Part model, mm, in its own coordinate system. A direction names the side the tool comes from. Coordinates: 2 decimals unless noted, no trailing zeros. Loops run counter-clockwise (first coordinate to the right, second up) from the corner with the lowest first, then second, coordinate; pieces in that order, holes last. Notation, with made-up numbers: M 78,87.25 L 127,87.25 A22 cw 127,118.25 Z; hole C -4,64 d2. An arc over 180 degrees is marked long. Answer as CSV lines item,"result". Start each with the question number.
from build123d import *

# Parameters (mm, degrees)
SKETCH1_W                        = 38.1
SKETCH1_H                        = 19.05
BOSS_EXTRUDE1_DEPTH              = 27.94
SKETCH2_W                        = 8.89
SKETCH2_H                        = 19.05
CUT_EXTRUDE1_DEPTH               = 21.59
CUT_EXTRUDE2_DEPTH               = 31.75
F_43_0_089_DIAMETER_HOLE1_D      = 2.2606
F_51_0_067_DIAMETER_HOLE1_REACH  = 52.943
F_51_0_067_DIAMETER_HOLE1_BORE_R = 0.8509
FILLET1_R                        = 1.27
SKETCH11_R                       = 2.75
CUT_EXTRUDE3_DEPTH               = 2
SKETCH12_R                       = 2.159
SKETCH12_R_2                     = 2.1209
CUT_EXTRUDE4_DEPTH               = 2.54


with BuildPart() as part:
    # Sketch1 → Boss-Extrude1 (new body)
    with BuildSketch(Plane.XY):
        with Locations((19.05, 9.525)):
            Rectangle(SKETCH1_W, SKETCH1_H)
    extrude(amount=BOSS_EXTRUDE1_DEPTH)

    # Sketch2 → Cut-Extrude1 (cut)
    with BuildSketch(Plane.XY.offset(27.94)):
        with Locations((4.445, 9.525)):
            Rectangle(SKETCH2_W, SKETCH2_H)
        with Locations((33.655, 9.525)):
            Rectangle(SKETCH2_W, SKETCH2_H)
    extrude(amount=-CUT_EXTRUDE1_DEPTH, mode=Mode.SUBTRACT)

    # Sketch4 → Cut-Extrude2 (cut)
    with BuildSketch(Plane(origin=(0, 19.05, 0), x_dir=(1, 0, 0), z_dir=(0, 1, 0))):
        with BuildLine():
            Line((13.66521077, -14.965662769), (19.05, -6.35))
            Line((19.05, -6.35), (24.43478923, -14.965662769))
            ThreePointArc((24.43478923, -14.965662769), (19.05, -24.681156038), (13.66521077, -14.965662769))
        make_face()
    extrude(amount=-CUT_EXTRUDE2_DEPTH, mode=Mode.SUBTRACT)

    # #43 (0.089) Diameter Hole1 (through all)
    with Locations(Plane.XY.offset(6.35)):
        with Locations((3.81, 9.525), (34.29, 9.525)):
            Hole(F_43_0_089_DIAMETER_HOLE1_D / 2)

    # #51 (0.067) Diameter Hole1 bore → #51 (0.067) Diameter Hole1 (cut, up to next)
    with BuildSketch(Plane.XY.offset(27.94), mode=Mode.PRIVATE) as f_51_0_067_diameter_hole1_sk1:
        with Locations((19.05, 8.89)):
            Circle(F_51_0_067_DIAMETER_HOLE1_BORE_R)
    f_51_0_067_diameter_hole1_tool1 = extrude(f_51_0_067_diameter_hole1_sk1.sketch, amount=-F_51_0_067_DIAMETER_HOLE1_REACH, mode=Mode.PRIVATE) & part.part
    add(f_51_0_067_diameter_hole1_tool1.solids().sort_by_distance((19.05, 8.89, 27.94))[0], mode=Mode.SUBTRACT)

    # Fillet1
    fillet1_edges = [part.edges().sort_by_distance(p)[0] for p in [
        (19.05, 0, 27.94),
        (0, 19.05, 3.175),
        (0, 0, 3.175),
        (0, 9.525, 6.35),
        (4.445, 19.05, 6.35),
        (8.89, 9.525, 6.35),
        (8.89, 19.05, 17.145),
        (4.445, 0, 6.35),
        (8.89, 0, 17.145),
        (8.89, 9.525, 27.94),
        (19.05, 19.05, 27.94),
        (38.1, 19.05, 3.175),
        (38.1, 0, 3.175),
        (38.1, 9.525, 6.35),
        (33.655, 0, 6.35),
        (29.21, 9.525, 6.35),
        (29.21, 0, 17.145),
        (33.655, 19.05, 6.35),
        (29.21, 19.05, 17.145),
        (29.21, 9.525, 27.94),
        (19.05, 9.525, 6.35),
    ]]
    fillet(fillet1_edges, radius=FILLET1_R)

    # Sketch11 → Cut-Extrude3 (cut)
    with BuildSketch(Plane(origin=(0, 0, 0), x_dir=(-1, 0, 0), z_dir=(0, 0, -1))):
        with Locations((-19.05, 9.525)):
            Circle(SKETCH11_R)
    extrude(amount=-CUT_EXTRUDE3_DEPTH, mode=Mode.SUBTRACT)

    # Sketch12 → Cut-Extrude4 (cut)
    with BuildSketch(Plane.XY.offset(6.35)):
        with Locations((3.81, 9.525)):
            Circle(SKETCH12_R)
        with Locations((34.29, 9.525)):
            Circle(SKETCH12_R_2)
    extrude(amount=-CUT_EXTRUDE4_DEPTH, mode=Mode.SUBTRACT)


solid = part.part
Q1. Flat gauge pins, fed straight in: P1, Ø5, axis at y = 10, z = 17.5, coming from the +X side; P2, Ø4.5, axis at x = 4.5, y = 10, coming from the +Z side; P3, Ø8.5, axis at y = 6.5, z = 14.5, coming from the -X side. Where does each tip first touch, or does it go through?
Q2. Wall check: L1, parallel to X at y = 8.89, z = 25.8; L2, parallel to Y at x = 3.81, z = 2; L3, parallel to Z at x = 32, y = 7.5. Give the ranges that are in metal, low to high.
Q3. Slice it at C-C, the plane x = 3.81. Write the cut outline in (y, z), and give its area (3 significant figures).
Q4. Slice it at B-B, the plane z = 12.75. Write the cut outline in (x, y), and give its area (3 significant figures).
Q5. Two-plate mould, pull along Y, no slides. Class faces 1 (the face through (9.272, 18.688, 17.012)), 2 (the face through (0.362, 9.641, 5.968)), 3 (the face through (32.17, 9.62, 5.1)), 4 (the face through (19, 10, 2)): +Y half, -Y half, draft (parallel to the pull), parting line (faces both ways), or undercut.
Q6. Slice it at A-A, the plane x = 19.05. Write the cut outline in (y, z) (3 decimals).
Q7. Tool access for faces 5 (the face through (29.21, 9, 17)), 6 (the face through (33.699, 18.688, 5.968)), 7 (the face through (35.2, 8.6, 3.81)), 8 (the face through (8.89, 9, 17)), 9 (the face through (9.272, 0.362, 17.012)): list every direction of +Z, -Z, +X, -X, +Y, -Y with a clear straight run to the whole face (end or side of a thin tool).
Q8. Slice it at D-D, the plane y = 14.25. Write the cut outline in (x, z).
Solved:
1,P1,"stops at x = 29.21"
1,P2,"stops at z = 6.35"
1,P3,"stops at x = 8.89"
2,L1,"x = 8.89 to 18.2, 19.9 to 29.21"
2,L2,"y = 0 to 8.39, 10.66 to 19.05"
2,L3,"z = 0 to 6.35"
3,outline,"M 0,0 L 8.39,0 L 8.39,3.81 L 7.37,3.81 L 7.37,6.35 L 1.27,6.35 A1.27 ccw 0,5.08 Z; M 10.66,0 L 19.05,0 L 19.05,5.08 A1.27 ccw 17.78,6.35 L 11.68,6.35 L 11.68,3.81 L 10.66,3.81 Z"
3,area,"101 mm2"
4,outline,"M 8.89,1.27 A1.27 ccw 10.16,0 L 15.05,0 L 15.05,19.05 L 10.16,19.05 A1.27 ccw 8.89,17.78 Z; M 23.05,0 L 27.94,0 A1.27 ccw 29.21,1.27 L 29.21,17.78 A1.27 ccw 27.94,19.05 L 23.05,19.05 Z"
4,area,"233 mm2"
5,face 1,"+Y half"
5,face 2,"draft"
5,face 3,"undercut"
5,face 4,"undercut"
6,outline,"M 0,0 L 6.775,0 L 6.775,2 L 12.275,2 L 12.275,0 L 19.05,0 L 19.05,7.476 L 0,7.476 Z; M 0,24.681 L 8.039,24.681 L 8.039,27.94 L 1.27,27.94 A1.27 ccw 0,26.67 Z; M 9.741,24.681 L 19.05,24.681 L 19.05,26.67 A1.27 ccw 17.78,27.94 L 9.741,27.94 Z"
7,face 5,"+Z, +X, +Y, -Y"
7,face 6,"+Z, +X, +Y"
7,face 7,"+Z"
7,face 8,"+Z, -X, +Y, -Y"
7,face 9,"+Z, -X, -Y"
8,outline,"M 0,0 L 38.1,0 L 38.1,5.08 A1.27 ccw 36.83,6.35 L 30.48,6.35 A1.27 cw 29.21,7.62 L 29.21,26.67 A1.27 ccw 27.94,27.94 L 10.16,27.94 A1.27 ccw 8.89,26.67 L 8.89,7.62 A1.27 cw 7.62,6.35 L 1.27,6.35 A1.27 ccw 0,5.08 Z; hole M 13.67,14.97 L 17.97,8.07 A1.27 ccw 20.13,8.07 L 24.43,14.97 A6.35 ccw long Z"
